The listing builds one solid part. Answer for the finished solid, in the listing's coordinates (mm). A direction names the side the tool comes from. Round coordinates to 2 decimals unless told otherwise and drop trailing zeros. Loops run counter-clockwise (first coordinate to the right, second up) from the corner with the lowest first, then second, coordinate; pieces in that order, holes last. Notation, with made-up numbers: (-31.75, -4) -> (13.25, -4) arc R23 ccw to (13.25, 28) -> close; hole circle Ø10 at (-32.75, 22). An arc over 180 degrees is marked (long way). Answer in a Markdown table with one row per item. Add a question column.
```python
from build123d import *

# Parameters (mm, degrees)
F1_DEPTH = 7.5
F2_R     = 1
F3_R     = 1.25
F4_DEPTH = 3
F5_DEPTH = 13


with BuildPart() as f1:
    # F0 (on Top) → F1 (new body)
    with BuildSketch(Plane.XY):
        with BuildLine():
            Line((-4.25, 4), (-1, 0))
            Line((-1, 0), (-1, 9))
            ThreePointArc((-1, 9), (0, 10), (1, 9))
            Line((1, 9), (1, 0))
            Line((1, 0), (4.25, 4))
            Line((4.25, 4), (2.5, 5))
            Line((2.5, 5), (2.5, 10))
            Line((2.5, 10), (10, 10))
            Line((10, 10), (10, 11))
            Line((10, 11), (-10, 11))
            Line((-10, 11), (-10, 10))
            Line((-10, 10), (-2.5, 10))
            Line((-2.5, 10), (-2.5, 5))
            Line((-2.5, 5), (-4.25, 4))
        make_face()
    extrude(amount=F1_DEPTH)

    # F2
    f2_edges = [f1.edges().sort_by_distance(p)[0] for p in [
        (2.5, 10, 3.75),
        (-2.5, 10, 3.75),
    ]]
    fillet(f2_edges, radius=F2_R)

    # F3 (on face) → F4 (join)
    with BuildSketch(Plane(origin=(0, 11, 0), x_dir=(-1, 0, 0), z_dir=(0, 1, 0))):
        with BuildLine():
            ThreePointArc((0, 0), (2.65165, 1.09835), (3.75, 3.75))
            ThreePointArc((3.75, 3.75), (2.65165, 6.40165), (0, 7.5))
            ThreePointArc((0, 7.5), (-3.75, 3.75), (0, 0))
        make_face()
        with Locations((0, 3.75)):
            Circle(F3_R, mode=Mode.SUBTRACT)
    extrude(amount=F4_DEPTH)

    # F3 (on face) → F5 (cut)
    with BuildSketch(Plane(origin=(0, 11, 0), x_dir=(-1, 0, 0), z_dir=(0, 1, 0))):
        with Locations((0, 3.75)):
            Circle(F3_R)
    extrude(amount=-F5_DEPTH, mode=Mode.SUBTRACT)


solid = f1.part
```
Item 1: Section D-D, the plane y = 13 is taken. Write down the section's boundary in (x, z).
Item 2: Consider L1, parallel to X at y = 8.5, z = 6.25; L2, parallel to Y at x = 8, z = 3.25; L3, parallel to X at y = 1.25, z = 5.25. Determine where each line is inside the solid, lowest interval first. Write a range as from..to.
Item 3: The mould has two halves that part along Y. Classify faces 1 (the flat face through (3.39, 4.49, 3.7)), 2 (the flat face through (1, 14, 5)), 3 (the flat face through (-2, 7, 0)), 4 (the flat face through (2.5, 7, 4)): +Y half, -Y half, draft (parallel to the pull), parting line (faces both ways), or undercut.
Item 4: For faces 5 (the flat face through (-10, 10.5, 3.7)), 6 (the flat face through (-2.65, 2.03, 3.7)), 7 (the cylindrical face through (-2.801, 9.715, 3.802)), 8 (the cylindrical face through (2.785, 9.699, 3.802)), 9 (the flat face through (-1, 4, 6)), determine the directions among +Z, -Z, +X, -X, +Y, -Y from which every point of the face is accessible in a straight line to the end or side of a thin tool.
Item 5: Section A-A, the plane y = 5.5 is taken. Write down the section's boundary in (x, z).
Item 6: Flat-ended cylindrical pins translate along their axes: P1, Ø3.5, axis at y = 5.5, z = 5.5, coming from the +X side; P2, Ø4, axis at x = 4, z = 2.5, coming from the +Y side; P3, Ø1, axis at y = 8.5, z = 1.5, coming from the +X side; P4, Ø2, axis at x = -6.5, z = 4.5, coming from the -Y side. Find the tip coordinate at first contact, or state that the pin passes through.
Item 7: Section C-C, the plane z = 3.5 is taken. Write down the section's boundary in (x, y).
Item 8: Section B-B, the plane z = 6 is taken. Write down the section's boundary in (x, y).
Here are the results:
| question | item | result |
|---|---|---|
| 1 | outline | (-3.75, 3.75) arc R3.75 ccw to (0, 0) arc R3.75 ccw to (0, 7.5) arc R3.75 ccw to start; hole circle Ø2.5 at (0, 3.75) |
| 2 | L1 | x = -2.5..-1, 1..2.5 |
| 2 | L2 | y = 10..11 |
| 2 | L3 | x = -2.02..-1, 1..2.02 |
| 3 | face 1 | undercut |
| 3 | face 2 | +Y half |
| 3 | face 3 | draft |
| 3 | face 4 | undercut |
| 4 | face 5 | +Z, -Z, -X, +Y, -Y |
| 4 | face 6 | +Z, -Z, -X, -Y |
| 4 | face 7 | +Z, -Z, -X |
| 4 | face 8 | +Z, -Z, +X |
| 4 | face 9 | +Z, -Z, -Y |
| 5 | outline | (-2.5, 0) -> (-1, 0) -> (-1, 3) arc R1.25 cw to (-1, 4.5) -> (-1, 7.5) -> (-2.5, 7.5) -> close; (1, 0) -> (2.5, 0) -> (2.5, 7.5) -> (1, 7.5) -> (1, 4.5) arc R1.25 cw to (1, 3) -> close |
| 6 | P1 | stops at x = 4.25 |
| 6 | P2 | stops at y = 14 |
| 6 | P3 | stops at x = 2.5 |
| 6 | P4 | stops at y = 10 |
| 7 | outline | (-10, 10) -> (-3.5, 10) arc R1 cw to (-2.5, 9) -> (-2.5, 5) -> (-4.25, 4) -> (-1.22, 0.28) -> (-1.22, 14) -> (-3.74, 14) -> (-3.74, 11) -> (-10, 11) -> close; (1.22, 0.28) -> (4.25, 4) -> (2.5, 5) -> (2.5, 9) arc R1 cw to (3.5, 10) -> (10, 10) -> (10, 11) -> (3.74, 11) -> (3.74, 14) -> (1.22, 14) -> close |
| 8 | outline | (-10, 10) -> (-3.5, 10) arc R1 cw to (-2.5, 9) -> (-2.5, 5) -> (-4.25, 4) -> (-1, 0) -> (-1, 9) arc R1 cw to (1, 9) -> (1, 0) -> (4.25, 4) -> (2.5, 5) -> (2.5, 9) arc R1 cw to (3.5, 10) -> (10, 10) -> (10, 11) -> (3, 11) -> (3, 14) -> (-3, 14) -> (-3, 11) -> (-10, 11) -> close |
